Answer from the drawing. Dimensions are ordinates in mm from the lowest x, y and z of the part. A direction names the side the tool comes from. Coordinates: 2 decimals unless noted, no trailing zeros. Write each loop counter-clockwise with the first axis right and the second up, starting at its lowest first coordinate (ties: lowest second). Pieces come first, ordered by that corner, then holes. Notation, with made-up numbers: (1, 65.5) - (24, 65.5) arc R23 cw to (24, 101.5) - close; hole circle Ø2 at (80, 12). An arc over 180 degrees is marked (long way). Return JSON: item names as keys, results as strings.
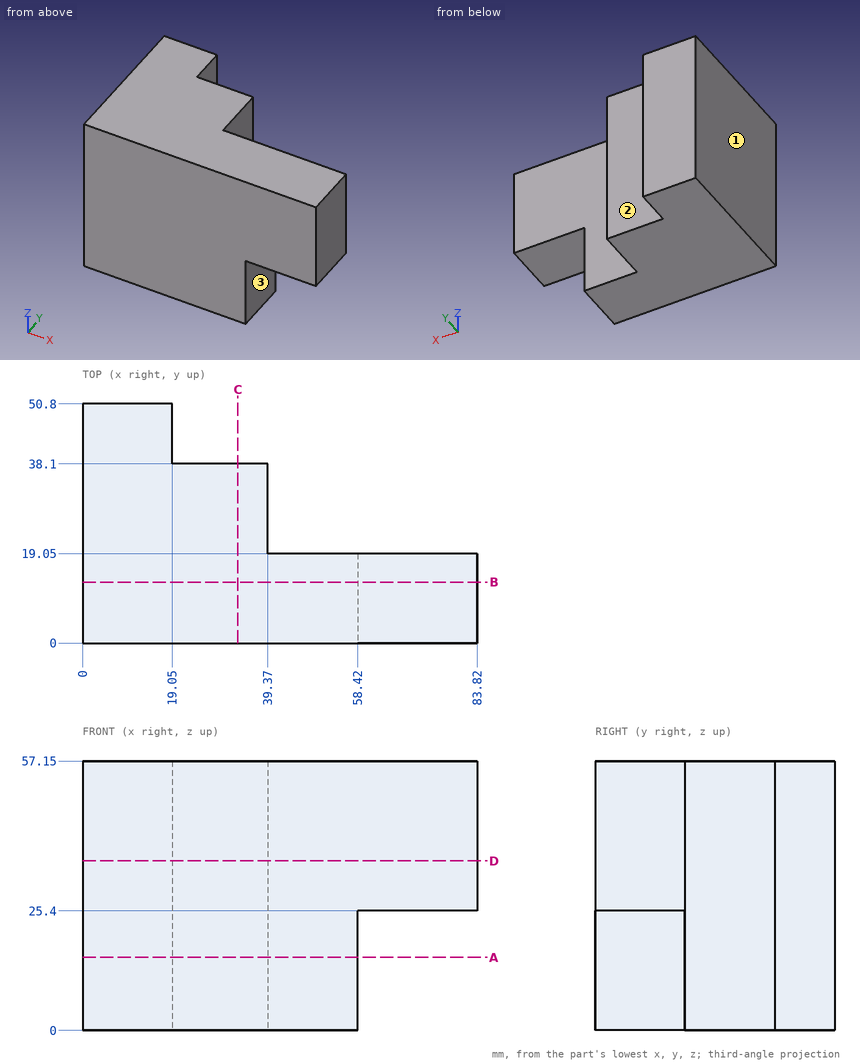
(1) Straight lines are drawn through the part: line 1 (Y direction, x = 20, z = 15); line 2 (Y direction, x = 44, z = 19). For each, find the intervals that lie inside material, in ascending order. Write a range as from..to.
Answer:
{"line 1": "0..38.1", "line 2": "0..19.05"}
(2) Flat-ended cylindrical pins translate along their axes: P1, Ø1.5, axis at x = 34, z = 24, coming from the +Y side; P2, Ø6.5, axis at y = 44, z = 36.5, coming from the +X side; P3, Ø9.5, axis at y = 9.5, z = 14.5, coming from the +X side; P4, Ø10, axis at x = 68, z = 15.5, coming from the +Y side. Find the tip coordinate at first contact, or state that the pin passes through.
Answer:
{"P1": "y = 38.1", "P2": "x = 19.05", "P3": "x = 58.42", "P4": "through"}
(3) A cutting plane is placed at B-B (y = 13). Determine the outline of the cut face in (x, z), and give its area (3 significant figures).
Answer:
{"outline": "(0, 0) - (58.42, 0) - (58.42, 25.4) - (83.82, 25.4) - (83.82, 57.15) - (0, 57.15) - close", "area": "4,150 mm²"}
(4) A cutting plane is placed at D-D (z = 36). Determine the outline of the cut face in (x, y), and give its area (3 significant figures).
Answer:
{"outline": "(0, 0) - (83.82, 0) - (83.82, 19.05) - (39.37, 19.05) - (39.37, 38.1) - (19.05, 38.1) - (19.05, 50.8) - (0, 50.8) - close", "area": "2,590 mm²"}
(5) A cutting plane is placed at C-C (x = 33). Determine the outline of the cut face in (y, z).
Answer:
{"outline": "(0, 0) - (38.1, 0) - (38.1, 57.15) - (0, 57.15) - close"}
(6) A cutting plane is placed at A-A (z = 15.5). Determine the outline of the cut face in (x, y), and give its area (3 significant figures).
Answer:
{"outline": "(0, 0) - (58.42, 0) - (58.42, 19.05) - (39.37, 19.05) - (39.37, 38.1) - (19.05, 38.1) - (19.05, 50.8) - (0, 50.8) - close", "area": "2,100 mm²"}
(7) Which of the six approach directions +Z, -Z, +X, -X, +Y, -Y give full straight-line access (tool end or side, diameter ignored) to the marked faces 1, 2 and 3?
Answer:
{"face 1": "+Z, -Z, -X, +Y, -Y", "face 2": "+Z, -Z, +X, +Y", "face 3": "-Z, +X, +Y, -Y"}
